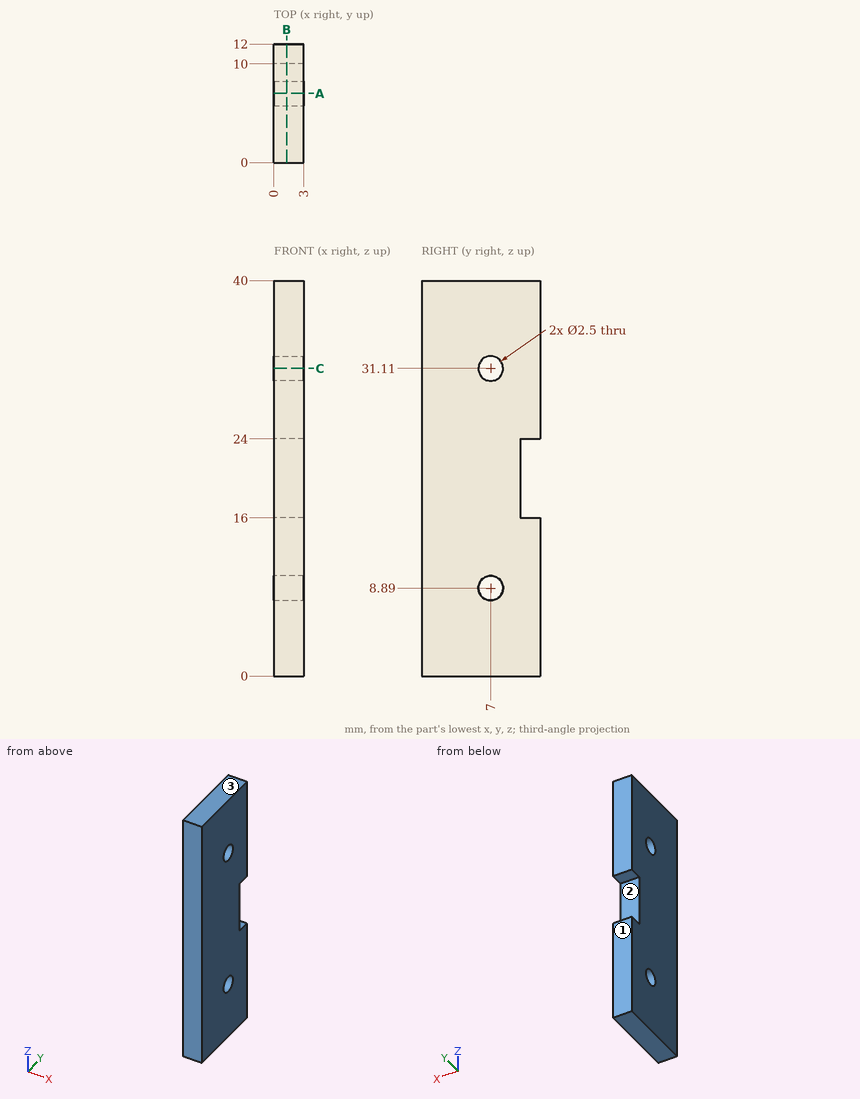
Could you check a few things on this drawing? It's one solid part, dimensions in mm from its lowest x, y, z. Coordinates: 2 decimals unless noted, no trailing zeros. Order: outer loops, then holes, each group sorted by start corner. A loop starts at its lowest first (then second) coordinate and runs counter-clockwise, first axis right, second up.
1) Imagine slicing it at A-A on y = 7. List the corners of the cut face in (x, z) for me.
2) We'd pull the mould along Z, two halves only. Please class the marked faces 1, 2 and 3: +Z half, -Z half, draft (parallel to the pull), parting line (faces both ways), or undercut.
3) Imagine slicing it at B-B on x = 1.3. List the corners of the cut face in (y, z) for me, and give its area (3 significant figures).
4) I need wall thicknesses on line 1 (Y direction, x = 1.3, z = 31.11); line 2 (Z direction, x = 2.25, y = 6); line 3 (Y direction, x = 1.3, z = 17.5). Which ranges of each line are inside material? Lowest first, please.
5) Imagine slicing it at C-C on z = 31.11. List the corners of the cut face in (x, y) for me, and give its area (3 significant figures).
Response values:
1. outline: (0, 0) - (3, 0) - (3, 7.64) - (0, 7.64) - close; (0, 10.14) - (3, 10.14) - (3, 29.86) - (0, 29.86) - close; (0, 32.36) - (3, 32.36) - (3, 40) - (0, 40) - close
2. face 1: draft
2. face 2: undercut
2. face 3: +Z half
3. outline: (0, 0) - (12, 0) - (12, 16) - (10, 16) - (10, 24) - (12, 24) - (12, 40) - (0, 40) - close; hole circle Ø2.5 at (7, 8.89); hole circle Ø2.5 at (7, 31.11)
3. area: 454 mm2
4. line 1: y = 0 to 5.75, 8.25 to 12
4. line 2: z = 0 to 8.14, 9.64 to 30.36, 31.86 to 40
4. line 3: y = 0 to 10
5. outline: (0, 0) - (3, 0) - (3, 5.75) - (0, 5.75) - close; (0, 8.25) - (3, 8.25) - (3, 12) - (0, 12) - close
5. area: 28.5 mm2
